Work out the finished part from the listing and answer in its coordinate system (mm). Face numbers are marked on the shaded views. A direction names the side the tool comes from. Round coordinates to 2 decimals unless told otherwise and drop trailing zeros. Write each loop counter-clockwise with the first axis right and the second up, starting at its lowest first coordinate (ties: lowest second). Pieces come first, ordered by that corner, then holes. Notation, with made-up numbers: (39, -0.75) - (71, -0.75) arc R14 ccw to (71, 3.25) - close; hole circle Ø5 at (70, 78). An arc over 180 degrees is marked (long way). Write item = value, one per line. Start each with the question number.
from build123d import *

# Parameters (mm, degrees)
SKETCH032_AS_DRAWN_W                      = 36.96
SKETCH032_AS_DRAWN_H                      = 13
EXTRUDE030_DEPTH                          = 2
EXTRUDE030_ONTO_SKETCH032_ROLL_ANGLE      = -0.051214
EXTRUDE030_ONTO_SKETCH032_PITCH_ANGLE     = -0.005439
EXTRUDE030_ONTO_SKETCH032_PLACEMENT_ANGLE = 89.992627
SKETCH031_W                               = 37
SKETCH031_H                               = 2.5
EXTRUDE029_DEPTH                          = 120
SKETCH030_W                               = 56
SKETCH030_H                               = 13.5
EXTRUDE028_DEPTH                          = 41


with BuildPart() as sensorcuts:
    # Sketch032 as drawn → Extrude030 (new)
    with BuildSketch(Plane.XY):
        with Locations((-0.07, -91)):
            Rectangle(SKETCH032_AS_DRAWN_W, SKETCH032_AS_DRAWN_H)
    extrude(amount=EXTRUDE030_DEPTH)


with BuildPart() as sensorcuts_1:
    # Extrude030 onto Sketch032 roll: moved
    add(sensorcuts.part.rotate(Axis((0, 0, 0), (1, 0, 0)), EXTRUDE030_ONTO_SKETCH032_ROLL_ANGLE))


with BuildPart() as sensorcuts_2:
    # Extrude030 onto Sketch032 pitch: moved
    add(sensorcuts_1.part.rotate(Axis((0, 0, 0), (0, 1, 0)), EXTRUDE030_ONTO_SKETCH032_PITCH_ANGLE))


with BuildPart() as sensorcuts_3:
    # Extrude030 onto Sketch032 placement: moved
    add(sensorcuts_2.part.moved(Location((60.323514, 26.485707, 1.233372))).rotate(Axis((60.323514, 26.485707, 1.233372), (0, 0, 1)), EXTRUDE030_ONTO_SKETCH032_PLACEMENT_ANGLE))


with BuildPart() as sensorcuts_4:
    # Extrude030 placement: moved
    add(sensorcuts_3.part.moved(Location((0, 0, -4))))


with BuildPart() as extrude029:
    # Sketch031 → Extrude029 (new body)
    with BuildSketch(Plane.YZ.offset(56)):
        with Locations((26.412533, 0.5)):
            Rectangle(SKETCH031_W, SKETCH031_H)
    extrude(amount=EXTRUDE029_DEPTH)


with BuildPart() as band002:
    # Sketch030 → Extrude028 (new body)
    with BuildSketch(Plane.XZ.offset(-6)):
        Polygon((175, 3.5), (58, 3.5), (58, 15.5), (-2, 15.5), (-2, 0.5), (-122, 0.5), (-122, -2.5), (175, -2.5), align=None)
        with Locations((28, 6.75)):
            Rectangle(SKETCH030_W, SKETCH030_H, mode=Mode.SUBTRACT)
    extrude(amount=-EXTRUDE028_DEPTH)

    # Cut002: cut Extrude029
    add(extrude029.part, mode=Mode.SUBTRACT)

    # Cut003: cut sensorCuts
    add(sensorcuts_4.part, mode=Mode.SUBTRACT)


solid = band002.part
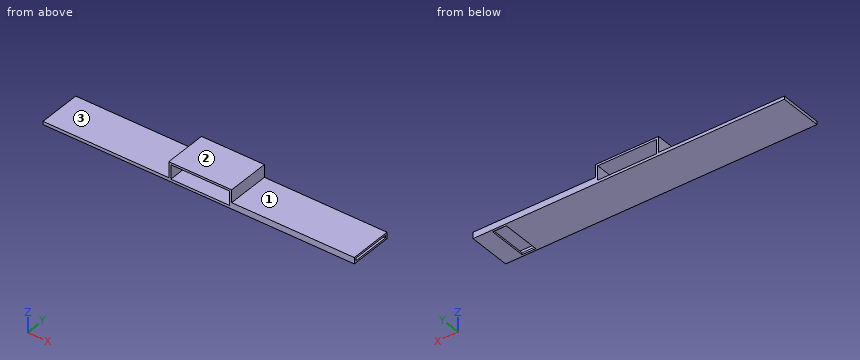
1. Find section D-D on x = 83. Give the vertices of the cut face in (y, z).
2. Find section C-C on y = 24. Give the vertices of the cut face in (x, z).
3. Find section B-B on z = 7.5. Give the vertices of the cut face in (x, y), plus the area to 3 significant figures.
4. Which of the six approach directions +Z, -Z, +X, -X, +Y, -Y give full straight-line access (tool end or side, diameter ignored) to the marked faces 1, 2 and 3?
5. Each of these flat-tipped pins is pushed along its axis until it touches: pin 1 (8 mm diameter, centred on y = 11.5, z = 11, fed in from -X); pin 2 (5 mm diameter, centred on x = -48.5, y = 22, fed in from +Z); pin 3 (1 mm diameter, centred on y = 29.5, z = 11.5, fed in from +X). Where does it stop, or does it pass through?
6. Consider line 1 (Z direction, x = 103, y = 22); line 2 (X direction, y = 27, z = 4); line 3 (Z direction, x = 13, y = 16). Determine where each line is inside the solid, lowest interval first.
7. Find section A-A on x = 46.5. Give the vertices of the cut face in (y, z).
Answer key:
q1.outline = (6, -2.5) - (47, -2.5) - (47, 3.5) - (6, 3.5) - close; hole (7.91, -0.75) - (44.91, -0.75) - (44.91, 1.75) - (7.91, 1.75) - close
q2.outline = (-122, -2.5) - (144.82, -2.5) - (144.82, -0.75) - (56, -0.75) - (56, 0) - (0, 0) - (0, 13.5) - (56, 13.5) - (56, 1.75) - (175, 1.75) - (175, 3.5) - (58, 3.5) - (58, 15.5) - (-2, 15.5) - (-2, 0.5) - (-122, 0.5) - close; (157.82, -2.5) - (175, -2.5) - (175, -0.75) - (157.82, -0.75) - close
q3.outline = (-2, 6) - (0, 6) - (0, 47) - (-2, 47) - close; (56, 6) - (58, 6) - (58, 47) - (56, 47) - close
q3.area = 164 mm²
q4.face_1 = +Z, +X, +Y, -Y
q4.face_2 = +Z, +X, -X, +Y, -Y
q4.face_3 = +Z, -X, +Y, -Y
q5.pin_1 = -2
q5.pin_2 = 0.5
q5.pin_3 = 58
q6.line_1 = -2.5 to -0.75, 1.75 to 3.5
q6.line_2 = -2 to 0, 56 to 58
q6.line_3 = -2.5 to 0, 13.5 to 15.5
q7.outline = (6, -2.5) - (47, -2.5) - (47, 0) - (6, 0) - close; (6, 13.5) - (47, 13.5) - (47, 15.5) - (6, 15.5) - close
